```python
from build123d import *

# Parameters (mm, degrees)
F1_DEPTH = 10
F2_R     = 3
F3_DEPTH = 10.001
F5_DEPTH = 4.7


with BuildPart() as f1:
    # F0 (on Top) → F1 (new body)
    with BuildSketch(Plane.XY):
        with BuildLine():
            ThreePointArc((-75, -5), (-72.071068, -12.071068), (-65, -15))
            Line((-65, -15), (65, -15))
            ThreePointArc((65, -15), (72.071068, -12.071068), (75, -5))
            Line((75, -5), (75, 5))
            ThreePointArc((75, 5), (72.071068, 12.071068), (65, 15))
            Line((65, 15), (-65, 15))
            ThreePointArc((-65, 15), (-72.071068, 12.071068), (-75, 5))
            Line((-75, 5), (-75, -5))
        make_face()
    extrude(amount=F1_DEPTH)

    # F2 (on face) → F3 (cut, through all)
    with BuildSketch(Plane.XY.offset(10)):
        with Locations((65, 0)):
            Circle(F2_R)
        with BuildLine():
            Line((53, 3.953533), (-67, 3.953533))
            ThreePointArc((-67, 3.953533), (-70.6, 0.353533), (-67, -3.246467))
            Line((-67, -3.246467), (53, -3.246467))
            ThreePointArc((53, -3.246467), (56.6, 0.353533), (53, 3.953533))
        make_face()
    extrude(amount=-F3_DEPTH, mode=Mode.SUBTRACT)

    # F4 (on face) → F5 (cut)
    with BuildSketch(Plane.XY.offset(10)):
        Polygon((62.754107, -3.89), (67.245893, -3.89), (69.491785, 0), (67.245893, 3.89), (62.754107, 3.89), (60.508215, 0), align=None)
    extrude(amount=-F5_DEPTH, mode=Mode.SUBTRACT)


solid = f1.part
```
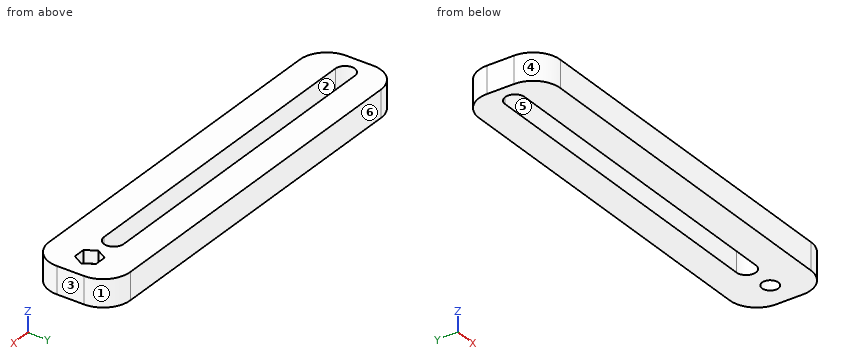
Can you work these out from the model? Positions are in its coordinate system, mm. Face numbers are marked on the shaded views. A direction names the side the tool comes from. Coordinates: 2 decimals unless noted, no trailing zeros. Loops run counter-clockwise (first coordinate to the right, second up) from the corner with the lowest first, then second, coordinate; pieces in that order, holes last. Notation, with made-up numbers: (-6.5, 7) - (30.5, 7) arc R33 ccw to (30.5, 36) - close; hole circle Ø8 at (31.25, 34.5). An arc over 180 degrees is marked (long way). Answer as CSV lines item,"result". Start each with the question number.
1) I need wall thicknesses on line 1 (Y direction, x = 25.5, z = 0.5); line 2 (Y direction, x = 65, z = 2.35); line 3 (X direction, y = -1.5, z = 4.25). Which ranges of each line are inside material? Lowest first, please. Write a range as from..to.
2) Suppose I cut it at C-C (z = 3). Please give me the cut outline in (x, y).
3) Thinking about a two-plate mould opening in Y: for the marked faces 3, 4, 5 and 6, which applies, pulls with the +Y half, pulls with the -Y half, needs draft (parallel to the pull), parting line crosses it, or undercut?
4) Suppose I cut it at A-A (z = 8.5). Please give me the cut outline in (x, y), plus the area to 3 significant figures.
5) Which directions (+Z, -Z, +X, -X, +Y, -Y) give clear straight access to the entire face, cutting with the end or side of a thin tool? Please do the marked faces 1 and 2.
6) Suppose I cut it at B-B (x = 50). Please give me the cut outline in (y, z), plus the area to 3 significant figures.
7) For pin 1 (7 mm diameter, centred on x = 65, y = 0, fed in from +Z); pin 2 (1.5 mm diameter, centred on y = -7, z = 2.5, fed in from +X); pin 3 (1.5 mm diameter, centred on y = -11, z = 3, fed in from +X), each with a flat end and sliding along its axis, tell me the tip position at first contact or that it passes through.
Check result:
1,line 1,"y = -15..-3.25, 3.95..15"
1,line 2,"y = -15..-3, 3..15"
1,line 3,"x = -75..-70.09, 56.09..62.4, 67.6..75"
2,outline,"(-75, -5) arc R10 ccw to (-65, -15) - (65, -15) arc R10 ccw to (75, -5) - (75, 5) arc R10 ccw to (65, 15) - (-65, 15) arc R10 ccw to (-75, 5) - close; hole (-67, -3.25) - (53, -3.25) arc R3.6 ccw to (53, 3.95) - (-67, 3.95) arc R3.6 ccw to start; hole circle Ø6 at (65, 0)"
3,face 3,"needs draft"
3,face 4,"pulls with the -Y half"
3,face 5,"undercut"
3,face 6,"pulls with the +Y half"
4,outline,"(-75, -5) arc R10 ccw to (-65, -15) - (65, -15) arc R10 ccw to (75, -5) - (75, 5) arc R10 ccw to (65, 15) - (-65, 15) arc R10 ccw to (-75, 5) - close; hole (-67, -3.25) - (53, -3.25) arc R3.6 ccw to (53, 3.95) - (-67, 3.95) arc R3.6 ccw to start; hole (60.51, 0) - (62.75, -3.89) - (67.25, -3.89) - (69.49, 0) - (67.25, 3.89) - (62.75, 3.89) - close"
4,area,"3,460 mm²"
5,face 1,"+Z, -Z, +X, +Y"
5,face 2,"+Z, -Z"
6,outline,"(-15, 0) - (-3.25, 0) - (-3.25, 10) - (-15, 10) - close; (3.95, 0) - (15, 0) - (15, 10) - (3.95, 10) - close"
6,area,"228 mm²"
7,pin 1,"stops at z = 5.3"
7,pin 2,"stops at x = 74.92"
7,pin 3,"stops at x = 73.51"
